Source: three-view drawing plus pictorial views. Frame: mm from the lowest corner of the part. A direction names the side the tool comes from. Give positions to 0.01 mm unless a question says otherwise; leave off trailing zeros. Order: outer loops, then holes, each group sorted by start corner. A loop starts at its lowest first (then second) coordinate and runs counter-clockwise, first axis right, second up. Notation, with made-up numbers: (79.25, -39.5) -> (101.25, -39.5) arc R19 cw to (101.25, -12.5) -> close; hole circle Ø2 at (-34, 52.5). An arc over 180 degrees is marked (long way). Answer in a Markdown table with one row per item.
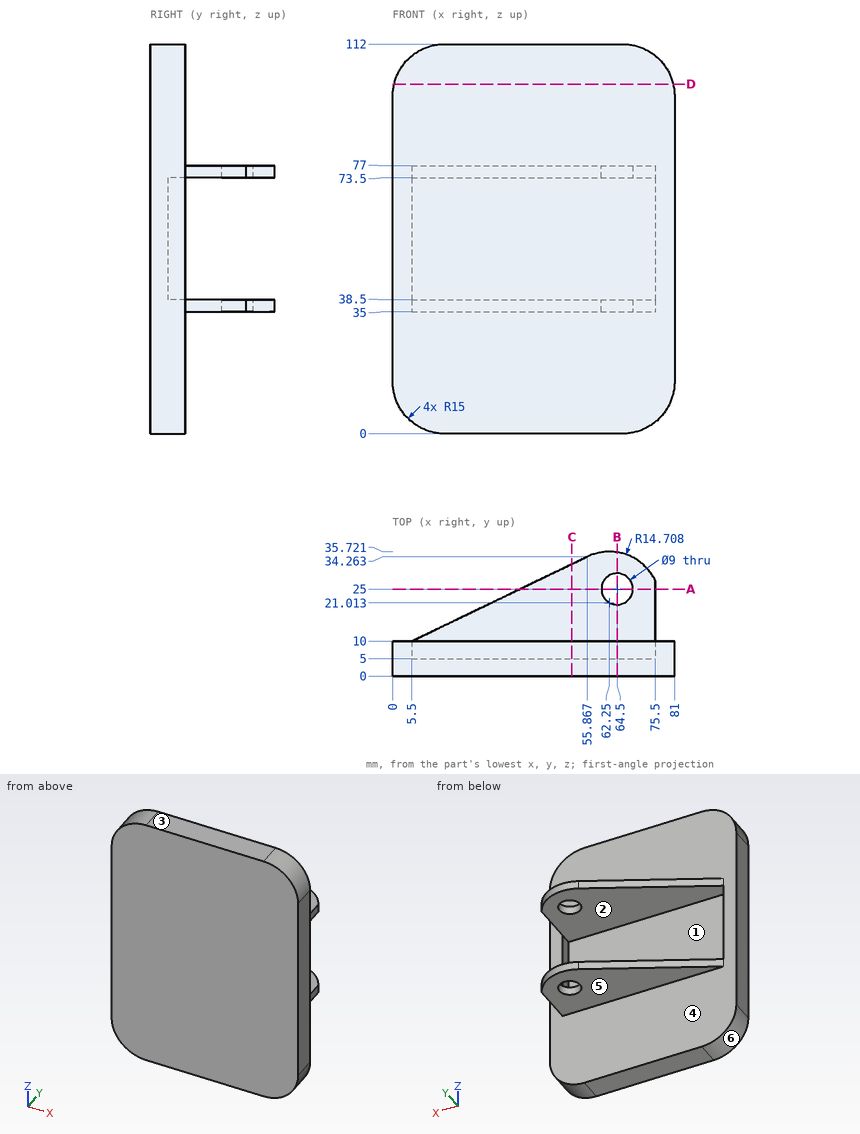
(1) Section query B-B (x = 64.5). Return the cut outline in (y, z), plus the area to 3 significant figures.
A:
| item | result |
|---|---|
| outline | (0, 0) -> (10, 0) -> (10, 35) -> (20.5, 35) -> (20.5, 38.5) -> (5, 38.5) -> (5, 73.5) -> (20.5, 73.5) -> (20.5, 77) -> (10, 77) -> (10, 112) -> (0, 112) -> close; (29.5, 35) -> (35.55, 35) -> (35.55, 38.5) -> (29.5, 38.5) -> close; (29.5, 73.5) -> (35.55, 73.5) -> (35.55, 77) -> (29.5, 77) -> close |
| area | 1,060 mm^2 |
(2) Section query C-C (x = 51.5). Return the cut outline in (y, z), plus the area to 3 significant figures.
A:
| item | result |
|---|---|
| outline | (0, 0) -> (10, 0) -> (10, 35) -> (32.16, 35) -> (32.16, 38.5) -> (5, 38.5) -> (5, 73.5) -> (32.16, 73.5) -> (32.16, 77) -> (10, 77) -> (10, 112) -> (0, 112) -> close |
| area | 1,100 mm^2 |
(3) Section query D-D (z = 100.5). Return the cut outline in (x, y) (1 decimal), plus the area to 3 significant figures.
A:
| item | result |
|---|---|
| outline | (0.4, 0) -> (80.6, 0) -> (80.6, 10) -> (0.4, 10) -> close |
| area | 802 mm^2 |
(4) Pull-direction query (Z, two-part tool) for the marked faces 1, 2, 3 and 4; classes: +Z half, -Z half, draft (parallel to the pull), parting line (faces both ways), or undercut.
A:
| item | result |
|---|---|
| face 1 | undercut |
| face 2 | undercut |
| face 3 | +Z half |
| face 4 | draft |
(5) Ray query, probe 1 along Z at (x, y) = (59, 16); probe 2 along Y at (x, z) = (24, 19); probe 3 along Y at (x, z) = (64.5, 37). Return the intervals inside material, ascending.
A:
| item | result |
|---|---|
| probe 1 | z = 35 to 38.5, 73.5 to 77 |
| probe 2 | y = 0 to 10 |
| probe 3 | y = 0 to 20.5, 29.5 to 35.55 |
(6) Section query A-A (y = 25). Return the cut outline in (x, z), plus the area to 3 significant figures.
A:
| item | result |
|---|---|
| outline | (36.64, 35) -> (60, 35) -> (60, 38.5) -> (36.64, 38.5) -> close; (36.64, 73.5) -> (60, 73.5) -> (60, 77) -> (36.64, 77) -> close; (69, 35) -> (75.5, 35) -> (75.5, 38.5) -> (69, 38.5) -> close; (69, 73.5) -> (75.5, 73.5) -> (75.5, 77) -> (69, 77) -> close |
| area | 209 mm^2 |
(7) First-contact query: pin 1 Ø11.5 at (x, y) = (64.5, 25) entering from -Z; pin 2 Ø1 at (x, z) = (65.5, 81.5) entering from +Y; pin 3 Ø9 at (x, y) = (23.5, 17.5) entering from +Z. Flat tips, straight axial feed; report the tip coordinate or a pass-through.
A:
| item | result |
|---|---|
| pin 1 | stops at z = 35 |
| pin 2 | stops at y = 10 |
| pin 3 | stops at z = 77 |
(8) Access query for the marked faces 5 and 6. Directions: +Z, -Z, +X, -X, +Y, -Y. A direction counts if a zero-diameter tool reaches every point of the face in a straight line with its end or side. Return the directions, or none.
A:
| item | result |
|---|---|
| face 5 | -Z, +X, -X, +Y |
| face 6 | -Z, -X, +Y, -Y |
